Read the model definition and answer for the solid it produces. Units are mm, in the model's axes. Give positions to 0.01 mm unless a question says otherwise; leave off trailing zeros. Loops run counter-clockwise (first coordinate to the right, second up) from the corner with the lowest first, then second, coordinate; pieces in that order, holes last. Notation, with made-up numbers: (62, 53.25) -> (68, 53.25) arc R31 cw to (68, 92.25) -> close; hole circle Ø9 at (-24.75, 31.5). An arc over 180 degrees is marked (long way). Answer as CSV lines item,"result". Start each with the question number.
```python
from build123d import *

# Parameters (mm, degrees)
CROQUIS1_W               = 2
CROQUIS1_H               = 2
SALIENTE_EXTRUIR1_DEPTH  = 0.2
CROQUIS2_W               = 2.6
CROQUIS2_H               = 2.6
SALIENTE_EXTRUIR2_DEPTH  = 0.2
CROQUIS3_W               = 3.2
CROQUIS3_H               = 3.2
SALIENTE_EXTRUIR3_DEPTH  = 0.2
CROQUIS4_W               = 3.8
CROQUIS4_H               = 3.8
SALIENTE_EXTRUIR4_DEPTH  = 0.2
CROQUIS5_W               = 4.4
CROQUIS5_H               = 4.4
SALIENTE_EXTRUIR5_DEPTH  = 0.2
CROQUIS6_W               = 5
CROQUIS6_H               = 5
SALIENTE_EXTRUIR6_DEPTH  = 0.2
CROQUIS7_W               = 5.6
CROQUIS7_H               = 5.6
SALIENTE_EXTRUIR7_DEPTH  = 0.2
CROQUIS8_W               = 6.2
CROQUIS8_H               = 6.2
SALIENTE_EXTRUIR8_DEPTH  = 0.2
CROQUIS9_W               = 6.8
CROQUIS9_H               = 6.8
SALIENTE_EXTRUIR9_DEPTH  = 0.2
CROQUIS10_W              = 7.4
CROQUIS10_H              = 7.4
SALIENTE_EXTRUIR10_DEPTH = 0.2
CROQUIS11_W              = 16.4
CROQUIS11_H              = 15.4
SALIENTE_EXTRUIR11_DEPTH = 3
CROQUIS12_R              = 1
CORTAR_EXTRUIR1_DEPTH    = 16.4


with BuildPart() as part:
    # Croquis1 → Saliente-Extruir1 (new body)
    with BuildSketch(Plane(origin=(0, 0, 0), x_dir=(1, 0, 0), z_dir=(0, 1, 0))):
        with Locations((1, -1)):
            Rectangle(CROQUIS1_W, CROQUIS1_H)
    extrude(amount=SALIENTE_EXTRUIR1_DEPTH)

    # Croquis2 → Saliente-Extruir2 (add)
    with BuildSketch(Plane(origin=(0, 0.2, 0), x_dir=(1, 0, 0), z_dir=(0, 1, 0))):
        with Locations((1, -1)):
            Rectangle(CROQUIS2_W, CROQUIS2_H)
    extrude(amount=SALIENTE_EXTRUIR2_DEPTH)

    # Croquis3 → Saliente-Extruir3 (add)
    with BuildSketch(Plane(origin=(0, 0.4, 0), x_dir=(1, 0, 0), z_dir=(0, 1, 0))):
        with Locations((1, -1)):
            Rectangle(CROQUIS3_W, CROQUIS3_H)
    extrude(amount=SALIENTE_EXTRUIR3_DEPTH)

    # Croquis4 → Saliente-Extruir4 (add)
    with BuildSketch(Plane(origin=(0, 0.6, 0), x_dir=(1, 0, 0), z_dir=(0, 1, 0))):
        with Locations((1, -1)):
            Rectangle(CROQUIS4_W, CROQUIS4_H)
    extrude(amount=SALIENTE_EXTRUIR4_DEPTH)

    # Croquis5 → Saliente-Extruir5 (add)
    with BuildSketch(Plane(origin=(0, 0.8, 0), x_dir=(1, 0, 0), z_dir=(0, 1, 0))):
        with Locations((1, -1)):
            Rectangle(CROQUIS5_W, CROQUIS5_H)
    extrude(amount=SALIENTE_EXTRUIR5_DEPTH)

    # Croquis6 → Saliente-Extruir6 (add)
    with BuildSketch(Plane(origin=(0, 1, 0), x_dir=(1, 0, 0), z_dir=(0, 1, 0))):
        with Locations((1, -1)):
            Rectangle(CROQUIS6_W, CROQUIS6_H)
    extrude(amount=SALIENTE_EXTRUIR6_DEPTH)

    # Croquis7 → Saliente-Extruir7 (add)
    with BuildSketch(Plane(origin=(0, 1.2, 0), x_dir=(1, 0, 0), z_dir=(0, 1, 0))):
        with Locations((1, -1)):
            Rectangle(CROQUIS7_W, CROQUIS7_H)
    extrude(amount=SALIENTE_EXTRUIR7_DEPTH)

    # Croquis8 → Saliente-Extruir8 (add)
    with BuildSketch(Plane(origin=(0, 1.4, 0), x_dir=(1, 0, 0), z_dir=(0, 1, 0))):
        with Locations((1, -1)):
            Rectangle(CROQUIS8_W, CROQUIS8_H)
    extrude(amount=SALIENTE_EXTRUIR8_DEPTH)

    # Croquis9 → Saliente-Extruir9 (add)
    with BuildSketch(Plane(origin=(0, 1.6, 0), x_dir=(1, 0, 0), z_dir=(0, 1, 0))):
        with Locations((1, -1)):
            Rectangle(CROQUIS9_W, CROQUIS9_H)
    extrude(amount=SALIENTE_EXTRUIR9_DEPTH)

    # Croquis10 → Saliente-Extruir10 (add)
    with BuildSketch(Plane(origin=(0, 1.8, 0), x_dir=(1, 0, 0), z_dir=(0, 1, 0))):
        with Locations((1, -1)):
            Rectangle(CROQUIS10_W, CROQUIS10_H)
    extrude(amount=SALIENTE_EXTRUIR10_DEPTH)

    # Croquis11 → Saliente-Extruir11 (add)
    with BuildSketch(Plane(origin=(0, 2, 0), x_dir=(1, 0, 0), z_dir=(0, 1, 0))):
        with Locations((1.5, -1)):
            Rectangle(CROQUIS11_W, CROQUIS11_H)
    extrude(amount=SALIENTE_EXTRUIR11_DEPTH)

    # Croquis12 → Cortar-Extruir1 (cut, through all)
    with BuildSketch(Plane.XY.offset(8.7)):
        with Locations((7.7, 3.5)):
            Circle(CROQUIS12_R)
    extrude(amount=-CORTAR_EXTRUIR1_DEPTH, mode=Mode.SUBTRACT)


solid = part.part
```
(1) Find section D-D on x = -5.5. Write down the section's boundary in (y, z), then the cut area to 3 significant figures.
(2) Find section A-A on y = 3.5. Write down the section's boundary in (x, z), then the cut area to 3 significant figures.
(3) Find section B-B on x = 7.7. Write down the section's boundary in (y, z).
(4) Find section C-C on z = 5.5. Write down the section's boundary in (x, y).
(5) This flat-tipped pin is pushed along its axis until it touches: P1, Ø3.5, axis at x = 1, z = 1.5, coming from the -Y side. Where does it stop, or does it pass through?
(6) Find the intervals of material crossed by line 1 along Y through (x, z) = (7.7, -2.25); line 2 along Y through (x, z) = (-5.25, -4.75); line 3 along X through (y, z) = (3.3, 0.25), in increasing order. Write a range as from..to.
Answer block:
1,outline,"(2, -6.7) -> (5, -6.7) -> (5, 8.7) -> (2, 8.7) -> close"
1,area,"46.2 mm2"
2,outline,"(-6.7, -6.7) -> (6.7, -6.7) -> (6.7, 8.7) -> (-6.7, 8.7) -> close; (8.7, -6.7) -> (9.7, -6.7) -> (9.7, 8.7) -> (8.7, 8.7) -> close"
2,area,"222 mm2"
3,outline,"(2, -6.7) -> (2.5, -6.7) -> (2.5, 8.7) -> (2, 8.7) -> close; (4.5, -6.7) -> (5, -6.7) -> (5, 8.7) -> (4.5, 8.7) -> close"
4,outline,"(-6.7, 2) -> (9.7, 2) -> (9.7, 5) -> (-6.7, 5) -> close; hole circle Ø2 at (7.7, 3.5)"
5,P1,"stops at y = 0"
6,line 1,"y = 2..2.5, 4.5..5"
6,line 2,"y = 2..5"
6,line 3,"x = -6.7..6.72, 8.68..9.7"
